```python
from build123d import *

# Parameters (mm, degrees)
EXTRUDE_DEPTH = 3.3
SKETCH001_R   = 1.5
POCKET_DEPTH  = 3.301
PAD_DEPTH     = 1


with BuildPart() as part:
    # Sketch → Extrude (new body)
    with BuildSketch(Plane.XY):
        with BuildLine():
            ThreePointArc((3.5, 21.5), (0, 25), (-3.5, 21.5))
            Line((-3.5, 21.5), (-3.5, 19.691369))
            ThreePointArc((-3.5, 19.691369), (0, -20), (3.5, 19.691369))
            Line((3.5, 19.691369), (3.5, 21.5))
        make_face()
    extrude(amount=EXTRUDE_DEPTH)

    # Sketch001 → Pocket (cut, through all)
    with BuildSketch(Plane.XY.offset(3.3)):
        with Locations((0, 21.5)):
            Circle(SKETCH001_R)
    extrude(amount=-POCKET_DEPTH, mode=Mode.SUBTRACT)

    # Sketch002 → Pad (new body)
    with BuildSketch(Plane.XY.offset(3.3)):
        with BuildLine():
            ThreePointArc((-3.2, 9.765466), (0, -13.8), (3.2, 9.765466))
            Line((3.2, 9.765466), (3.2, 6.765466))
            ThreePointArc((-3.2, 6.765466), (0, -10.943698), (3.2, 6.765466))
            Line((-3.2, 9.765466), (-3.2, 6.765466))
        make_face()
        with BuildLine():
            ThreePointArc((1.5, 13.5), (0, 15), (-1.5, 13.5))
            Line((-1.5, 13.5), (-1.5, -5))
            ThreePointArc((-1.5, -5), (0, -6.5), (1.5, -5))
            Line((1.5, 13.5), (1.5, -5))
        make_face()
    extrude(amount=PAD_DEPTH)


solid = part.part
```
Verification items for the finished model (mm, model axes). A direction names the side the tool comes from. Coordinates: 2 decimals unless noted, no trailing zeros. Loops run counter-clockwise (first coordinate to the right, second up) from the corner with the lowest first, then second, coordinate; pieces in that order, holes last. Notation, with made-up numbers: (58, 4.5) -> (110, 4.5) arc R30 cw to (110, 31.5) -> close; hole circle Ø4 at (-5, 67.5). An arc over 180 degrees is marked (long way). Put each result on its own line as item: value.
1. Mould release check, pull along Y, two halves, no side actions. Record for faces 5 (the face through (-0.83, -19.983, 1.627)), 6 (the face through (-0.356, -10.937, 3.793)), 7 (the face through (-3.5, 21, 2)): pulls with the +Y half, pulls with the -Y half, needs draft (parallel to the pull), parting line crosses it, or undercut.
Result set:
face 5: parting line crosses it
face 6: undercut
face 7: needs draft
2. Section check A-A, the plane z = 3.8. Record the boundary of the cut face in (x, y), then the cut area to 3 significant figures.
Result set:
outline: (-3.2, 6.77) -> (-3.2, 9.77) arc R12 ccw (long way) to (3.2, 9.77) -> (3.2, 6.77) arc R9.14 cw (long way) to start; (-1.5, -5) arc R1.5 ccw to (1.5, -5) -> (1.5, 13.5) arc R1.5 ccw to (-1.5, 13.5) -> close
area: 234 mm^2
3. Section check D-D, the plane z = 1.25. Record the boundary of the cut face in (x, y).
Result set:
outline: (-3.5, 19.69) arc R20 ccw (long way) to (3.5, 19.69) -> (3.5, 21.5) arc R3.5 ccw to (-3.5, 21.5) -> close; hole circle Ø3 at (0, 21.5)
4. Section check C-C, the plane y = 22.5. Record the boundary of the cut face in (x, z), then the cut area to 3 significant figures.
Result set:
outline: (-3.35, 0) -> (-1.12, 0) -> (-1.12, 3.3) -> (-3.35, 3.3) -> close; (1.12, 0) -> (3.35, 0) -> (3.35, 3.3) -> (1.12, 3.3) -> close
area: 14.8 mm^2
5. Thickness scan on line 1 (X direction, y = -1.8, z = 3.7); line 2 (X direction, y = 4, z = 3.4); line 3 (Z direction, x = 4, y = -4). Record the ranges inside material, lowest first.
Result set:
line 1: x = -12 to -9.14, -1.5 to 1.5, 9.14 to 12
line 2: x = -10.51 to -7.07, -1.5 to 1.5, 7.07 to 10.51
line 3: z = 0 to 3.3
6. Section check B-B, the plane x = 0. Record the boundary of the cut face in (y, z).
Result set:
outline: (-20, 0) -> (20, 0) -> (20, 3.3) -> (15, 3.3) -> (15, 4.3) -> (-6.5, 4.3) -> (-6.5, 3.3) -> (-10.94, 3.3) -> (-10.94, 4.3) -> (-13.8, 4.3) -> (-13.8, 3.3) -> (-20, 3.3) -> close; (23, 0) -> (25, 0) -> (25, 3.3) -> (23, 3.3) -> close
7. Tool access check on faces 1 (the face through (-3.2, 8, 4)), 2 (the face through (0, -6.5, 3.8)), 3 (the face through (3.5, 21, 2)), 4 (the face through (0, 25, 2)). Record the directions out of +Z, -Z, +X, -X, +Y, -Y that give a thin tool (end or side, any length) a straight path to the whole face; none if there is none.
Result set:
face 1: +Z, +Y
face 2: +Z
face 3: +Z, -Z, +X, +Y
face 4: +Z, -Z, +Y
8. Gauge pin test, flat ends, axial feed: P1, Ø2, axis at x = -8, y = 18.5, coming from the +Z side; P2, Ø1.5, axis at y = 10, z = 2, coming from the -X side; P3, Ø0.8, axis at y = 7.5, z = 4, coming from the -X side; P4, Ø2.5, axis at x = 0, y = 21.5, coming from the +Z side. Record the tip position at first contact, or that the pin passes through.
Result set:
P1: stops at z = 3.3
P2: stops at x = -17.73
P3: stops at x = -8.05
P4: passes through
